Design review of the part built by this model. Coordinates are the model's own, in mm. Give positions to 0.01 mm unless a question says otherwise; leave off trailing zeros. Write each loop counter-clockwise with the first axis right and the second up, starting at its lowest first coordinate (ties: lowest second). Pieces come first, ordered by that corner, then holes. Notation, with made-up numbers: M -6.75,-32.5 L 9.25,-32.5 A21 ccw 9.25,0.5 Z; hole C -23,-31 d11. An arc over 180 degrees is marked long. Write each question's results on one line, items separated by ' | '. Start each with the question number.
from build123d import *

# Parameters (mm, degrees)
BOSS_EXTRUDE1_DEPTH = 3


with BuildPart() as part:
    # Sketch3 → Boss-Extrude1 (new body)
    with BuildSketch(Plane.XY.offset(-2)):
        Polygon((-331.826668729, 452.47886283), (-275.647209147, 408.586658554), (-291.038746031, 388.886389714), (-362.193866809, 444.47886283), (-427.432442284, 444.47886283), (-447.432442284, 460.10457536), (-447.432442284, 561.679955314), (-427.432442284, 561.679955314), (-427.432442284, 452.47886283), align=None)
    extrude(amount=-BOSS_EXTRUDE1_DEPTH)


solid = part.part
Q1. We need section A-A on z = -3.5. Write out the cut boundary in (x, y), and give its area (3 significant figures).
Q2. We need section B-B on y = 468.5. Write out the cut boundary in (x, z).
Q3. For pin 1 Ø1 at (x, z) = (-410, -4.5) entering from +Y; pin 2 Ø1.5 at (x, z) = (-406, -4) entering from -Y; pin 3 Ø1.5 at (y, z) = (487, -3.5) entering from +X, all flat-tipped, find the tip position at first contact; note any pin that passes through.
Q4. Wall thickness on line 1 along Y through (x, z) = (-375.5, -4.3); line 2 along X through (y, z) = (523.5, -3.6); line 3 along X through (y, z) = (410.5, -4.25): over which ranges is each line inside the solid? List them lowest first. Write a range as from..to.
Q5. We need section C-C on x = -406. Write out the cut boundary in (y, z), and give its area (3 significant figures).
Answer sheet:
1) outline: M -447.43,460.1 L -427.43,444.48 L -362.19,444.48 L -291.04,388.89 L -275.65,408.59 L -331.83,452.48 L -427.43,452.48 L -427.43,561.68 L -447.43,561.68 Z | area: 4,850 mm^2
2) outline: M -447.43,-5 L -427.43,-5 L -427.43,-2 L -447.43,-2 Z
3) pin 1: y = 452.48 | pin 2: y = 444.48 | pin 3: x = -427.43
4) line 1: 444.48..452.48 | line 2: -447.43..-427.43 | line 3: -318.7..-278.1
5) outline: M 444.48,-5 L 452.48,-5 L 452.48,-2 L 444.48,-2 Z | area: 24.0 mm^2
